from build123d import *

# Parameters (mm, degrees)
SKETCH1_R                   = 30
BASE_FLANGE1_DEPTH          = 4
M3_TAPPED_BASE_D            = 2.5
M3_TAPPED_MOTOR_D           = 3.4
M3_TAPPED_MOTOR_CSINK_D     = 6.3
M3_TAPPED_MOTOR_CSINK_ANGLE = 90
SKETCH10_R                  = 14
CUT_EXTRUDE1_DEPTH          = 43.614551505


# Sheet-metal steps are written as plain solids
with BuildPart() as part:
    # Sketch1 → Base-Flange1 (new body)
    with BuildSketch(Plane(origin=(0, 0, 0), x_dir=(1, 0, 0), z_dir=(0, 1, 0))):
        with Locations(Location((0, 0, 0), (0, 0, 270))):
            Circle(SKETCH1_R)
    extrude(amount=-BASE_FLANGE1_DEPTH)

    # M3 Tapped base (through all)
    with Locations(Plane(origin=(0, 0, 0), x_dir=(1, 0, 0), z_dir=(0, 1, 0))):
        with Locations((0, 25.5), (25.5, 0), (0, -25.5), (-25.5, 0)):
            Hole(M3_TAPPED_BASE_D / 2)

    # M3 Tapped motor (through all)
    with Locations(Plane.XZ.offset(4)):
        with Locations((-15.5, -15.5), (15.5, 15.5), (-15.5, 15.5), (15.5, -15.5)):
            CounterSinkHole(M3_TAPPED_MOTOR_D / 2, M3_TAPPED_MOTOR_CSINK_D / 2, counter_sink_angle=M3_TAPPED_MOTOR_CSINK_ANGLE)

    # Sketch10 → Cut-Extrude1 (cut, through all)
    with BuildSketch(Plane(origin=(0, -4, 0), x_dir=(-1, 0, 0), z_dir=(0, -1, 0))):
        with Locations(Location((0, 0, 0), (0, 0, 90))):
            Circle(SKETCH10_R)
    extrude(amount=-CUT_EXTRUDE1_DEPTH, mode=Mode.SUBTRACT)


solid = part.part
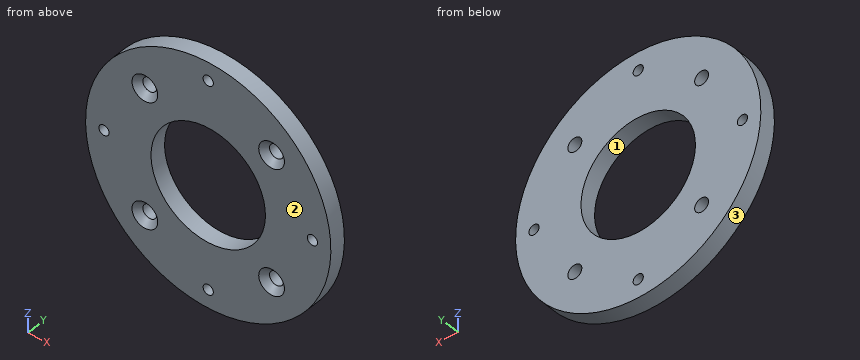
Part model, mm, in its own coordinate system. Face numbers are marked on the shaded views. Give positions to 0.01 mm unless a question says otherwise; leave off trailing zeros. Loops run counter-clockwise (first coordinate to the right, second up) from the corner with the lowest first, then second, coordinate; pieces in that order, holes last. Notation, with made-up numbers: (79, 86) -> (119, 86) arc R14 cw to (119, 105) -> close; hole circle Ø9 at (84, 4). An arc over 180 degrees is marked (long way). Write each question's results on one line, items separated by ' | '. Start each with the question number.
Q1. Band-saw the part on A-A on x = 0. List the corners of the cut face in (y, z).
Q2. Band-saw the part on D-D on z = -9.5. List the corners of the cut face in (x, y).
Q3. Wall check: L1, parallel to Z at x = -15.5, y = -1.55; L2, parallel to Z at x = 1, y = -1.2. Give the ranges that are in metal, low to high.
Q4. Pin check, flat tips, straight feed: P1, Ø1.5, axis at x = 3.5, y = -2.5, coming from the -Z side; P2, Ø5.5, axis at x = 15.5, z = -15.5, coming from the -Y side. Stop position of each tip, or through.
Q5. Pull direction X, two halves, no side cores. Call the marked faces 1, 2 and 3: +X half, -X half, draft (parallel to the pull), parting line (faces both ways), or undercut.
Q6. Band-saw the part on C-C on z = 0. List the corners of the cut face in (x, y).
Q7. Band-saw the part on B-B on y = -0.7. Count the separate pieces of the cut face and the enclosed holes in it, plus the area to 3 significant figures.
Results are:
1) outline: (-4, -30) -> (0, -30) -> (0, -26.75) -> (-4, -26.75) -> close; (-4, -24.25) -> (0, -24.25) -> (0, -14) -> (-4, -14) -> close; (-4, 14) -> (0, 14) -> (0, 24.25) -> (-4, 24.25) -> close; (-4, 26.75) -> (0, 26.75) -> (0, 30) -> (-4, 30) -> close
2) outline: (-28.46, -4) -> (-10.28, -4) -> (-10.28, 0) -> (-28.46, 0) -> close; (10.28, -4) -> (28.46, -4) -> (28.46, 0) -> (10.28, 0) -> close
3) L1: z = -25.69 to -17.2, -13.8 to 13.8, 17.2 to 25.69 | L2: z = -29.98 to -26.25, -24.75 to -13.96, 13.96 to 24.75, 26.25 to 29.98
4) P1: stops at z = -29.87 | P2: stops at y = -3.6
5) face 1: undercut | face 2: draft | face 3: parting line
6) outline: (-30, -4) -> (-26.75, -4) -> (-26.75, 0) -> (-30, 0) -> close; (-24.25, -4) -> (-14, -4) -> (-14, 0) -> (-24.25, 0) -> close; (14, -4) -> (24.25, -4) -> (24.25, 0) -> (14, 0) -> close; (26.75, -4) -> (30, -4) -> (30, 0) -> (26.75, 0) -> close
7) separate pieces: 1 | enclosed holes: 9 | area: 2,160 mm²
